```python
from build123d import *

# Parameters (mm, degrees)
SKETCH1_R           = 7.5
BOSS_EXTRUDE1_DEPTH = 10


with BuildPart() as part:
    # Sketch1 → Boss-Extrude1 (new body)
    with BuildSketch(Plane(origin=(0, 0, 0), x_dir=(0, 0, -1), z_dir=(1, 0, 0))):
        with BuildLine():
            Line((-25, 0), (25, 0))
            Line((25, 0), (25, 177.43174))
            ThreePointArc((25, 177.43174), (0, 202.43174), (-25, 177.43174))
            Line((-25, 177.43174), (-25, 0))
        make_face()
        with Locations((0, 95.2901012)):
            Circle(SKETCH1_R, mode=Mode.SUBTRACT)
        with Locations((0, 177.43174)):
            Circle(SKETCH1_R, mode=Mode.SUBTRACT)
    extrude(amount=BOSS_EXTRUDE1_DEPTH)


solid = part.part
```
Can you work these out from the model? Positions are in its coordinate system, mm. Coordinates: 2 decimals unless noted, no trailing zeros. Loops run counter-clockwise (first coordinate to the right, second up) from the corner with the lowest first, then second, coordinate; pieces in that order, holes last. Notation, with made-up numbers: M 11,79 L 62,79 A27 cw 62,113 Z; hole C -34,89 d7. An arc over 180 degrees is marked long. Put each result on its own line as item: value. Start each with the question number.
(1) We'd pull the mould along Y, two halves only. Please class faces 1 (the face through (4.93, 184.868, 0.976)), 2 (the face through (5, 87, -25)), 3 (the face through (4.93, 102.726, 0.976)), 4 (the face through (4.93, 202.426, -0.55)): +Y half, -Y half, draft (parallel to the pull), parting line (faces both ways), or undercut.
(2) Will these pins go through, and if not, where does the flat tip stop? pin 1 Ø2 at (x, z) = (8.5, 11.5) entering from +Y; pin 2 Ø3 at (x, z) = (6, 4.5) entering from +Y; pin 3 Ø1 at (x, z) = (2, -14.5) entering from +Y.
(3) Imagine slicing it at C-C on x = 7. List the corners of the cut face in (y, z) for me, and give its area (3 significant figures).
(4) Imagine slicing it at A-A on z = 0. List the corners of the cut face in (x, y) for me.
(5) I need wall thicknesses on probe 1 along Y at (x, z) = (4.5, 0); probe 2 along Y at (x, z) = (2, 1); probe 3 along Z at (x, y) = (2, 93). Which ranges of each line are inside material? Lowest first, please.
(6) Imagine slicing it at B-B on y = 89.5. List the corners of the cut face in (x, z) for me, and give its area (3 significant figures).
(7) Imagine slicing it at D-D on y = 180.5. List the corners of the cut face in (x, z) for me, and give its area (3 significant figures).
Worked answers:
1. face 1: undercut
1. face 2: draft
1. face 3: undercut
1. face 4: +Y half
2. pin 1: stops at y = 200.12
2. pin 2: stops at y = 202.25
2. pin 3: stops at y = 198.14
3. outline: M 0,-25 L 177.43,-25 A25 ccw 177.43,25 L 0,25 Z; hole C 95.29,0 d15; hole C 177.43,0 d15
3. area: 9,500 mm2
4. outline: M 0,0 L 10,0 L 10,87.79 L 0,87.79 Z; M 0,102.79 L 10,102.79 L 10,169.93 L 0,169.93 Z; M 0,184.93 L 10,184.93 L 10,202.43 L 0,202.43 Z
5. probe 1: y = 0 to 87.79, 102.79 to 169.93, 184.93 to 202.43
5. probe 2: y = 0 to 87.86, 102.72 to 170, 184.86 to 202.41
5. probe 3: z = -25 to -7.14, 7.14 to 25
6. outline: M 0,-25 L 10,-25 L 10,-4.77 L 0,-4.77 Z; M 0,4.77 L 10,4.77 L 10,25 L 0,25 Z
6. area: 405 mm2
7. outline: M 0,-24.81 L 10,-24.81 L 10,-6.84 L 0,-6.84 Z; M 0,6.84 L 10,6.84 L 10,24.81 L 0,24.81 Z
7. area: 359 mm2
